For this review, take the finished solid that the model builds, in its own axes (mm). Face numbers are marked on the shaded views. Round coordinates to 2 decimals unless told otherwise and drop trailing zeros. Order: outer loops, then holes, each group sorted by start corner. A loop starts at its lowest first (then second) coordinate and runs counter-clockwise, first axis right, second up. Notation, with made-up numbers: M -24,85 L -1,85 A19 cw -1,89 Z; hole C 70,72.25 d8. An arc over 180 degrees is marked long. Use a Markdown table: item, result.
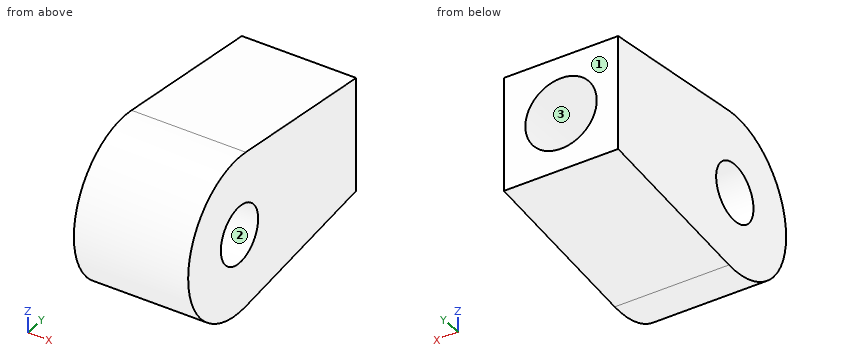
from build123d import *

# Parameters (mm, degrees)
IZIM1_R                     = 8
Y_KSEKLIK_EKSTR_ZYON1_DEPTH = 32
IZIM2_R                     = 10
KES_EKSTR_ZYON1_DEPTH       = 38


with BuildPart() as part:
    # Çizim1 → Yükseklik-Ekstrüzyon1 (new body)
    with BuildSketch(Plane(origin=(0, 0, 0), x_dir=(0, 0, -1), z_dir=(1, 0, 0))):
        with BuildLine():
            Line((-74.694543473, -11.370690029), (-68.859982056, 35.936369625))
            Line((-68.859982056, 35.936369625), (-36.859982056, 35.936369625))
            Line((-36.859982056, 35.936369625), (-31.001531459, -11.572016946))
            ThreePointArc((-31.001531459, -11.572016946), (-52.961351702, -36.063396833), (-74.694543473, -11.370690029))
        make_face()
        with Locations((-52.859982056, -14.063630375)):
            Circle(IZIM1_R, mode=Mode.SUBTRACT)
    extrude(amount=Y_KSEKLIK_EKSTR_ZYON1_DEPTH)

    # Çizim2 → Kes-Ekstrüzyon1 (cut)
    with BuildSketch(Plane(origin=(0, 35.936369625, 0), x_dir=(1, 0, 0), z_dir=(0, 1, 0))):
        with Locations(Location((16, -52.859982056, 0), (0, 0, 270))):
            Circle(IZIM2_R)
    extrude(amount=-KES_EKSTR_ZYON1_DEPTH, mode=Mode.SUBTRACT)


solid = part.part
Q1. Add section C-C (x = 8). Write out the cut boundary in (y, z), then the cut area to 3 significant figures.
Determined:
| item | result |
|---|---|
| outline | M -11.57,31 L 35.94,36.86 L 35.94,46.86 L -2.06,46.86 L -2.06,58.86 L 35.94,58.86 L 35.94,68.86 L -11.37,74.69 A22 ccw long Z; hole C -14.06,52.86 d16 |
| area | 2,010 mm^2 |
Q2. Add section B-B (y = -10). Write out the cut boundary in (x, z).
Determined:
| item | result |
|---|---|
| outline | M 0,31.2 L 32,31.2 L 32,45.97 L 0,45.97 Z; M 0,59.75 L 32,59.75 L 32,74.53 L 0,74.53 Z |
Q3. Clearance check with flat-ended pins moving along their axes: pin 1 (12 mm diameter, centred on x = 15, y = -29, fed in from -Z); pin 2 (1 mm diameter, centred on x = 25, y = 17, fed in from -Z); pin 3 (6 mm diameter, centred on x = 16.5, z = 54.5, fed in from +Y). State where each tip first meets the part, or that it passes through.
Determined:
| item | result |
|---|---|
| pin 1 | stops at z = 32.76 |
| pin 2 | stops at z = 34.46 |
| pin 3 | stops at y = -2.06 |
Q4. Wall thickness on line 1 along Z through (x, y) = (24.5, -14); line 2 along Z through (x, y) = (4.5, -14.5); line 3 along X through (y, z) = (0.5, 59): over which ranges is each line inside the solid? List them lowest first. Write a range as [from, to].
Determined:
| item | result |
|---|---|
| line 1 | z = [30.86, 44.86], [60.86, 74.86] |
| line 2 | z = [30.86, 44.87], [60.85, 74.86] |
| line 3 | x = [0, 8.11], [23.89, 32] |
Q5. Add section D-D (y = 3). Write out the cut boundary in (x, z).
Determined:
| item | result |
|---|---|
| outline | M 0,32.8 L 32,32.8 L 32,72.92 L 0,72.92 Z; hole C 16,52.86 d20 |
Q6. Draft analysis for pull direction Y (two halves, no side actions). For the marked faces 1, 2 and 3, state which applies: pulls with the +Y half, pulls with the -Y half, needs draft (parallel to the pull), parting line crosses it, or undercut.
Determined:
| item | result |
|---|---|
| face 1 | pulls with the +Y half |
| face 2 | undercut |
| face 3 | needs draft |
Q7. Add section A-A (z = 56). Write out the cut boundary in (x, y).
Determined:
| item | result |
|---|---|
| outline | M 0,-35.84 L 32,-35.84 L 32,-21.42 L 0,-21.42 Z; M 0,-6.71 L 32,-6.71 L 32,35.94 L 25.49,35.94 L 25.49,-2.06 L 6.51,-2.06 L 6.51,35.94 L 0,35.94 Z |
